```python
from build123d import *

# Parameters (mm, degrees)
SKETCH_1_R          = 1.65
EXTRUDE_1_DEPTH     = 3
SKETCH_3_W          = 62
SKETCH_3_H          = 11.5
EXTRUDE_2_DEPTH     = 3
FILLET_1_R          = 5
CUT_EXTRUDE_1_DEPTH = 10
SKETCH_4_R          = 4.5
SKETCH_4_R_2        = 1.75
EXTRUDE_3_DEPTH     = 3
FILLET_2_R          = 2
SKETCH_5_R          = 1.75
CUT_EXTRUDE_2_DEPTH = 3
SKETCH_6_OUTSIDE_W  = 115.11
SKETCH_6_OUTSIDE_H  = 116.61
CUT_EXTRUDE_4_DEPTH = 10
FILLET_3_R          = 5


with BuildPart() as part:
    # 草图1 → 凸台-拉伸1 (new body)
    with BuildSketch(Plane(origin=(0, 0, 0), x_dir=(1, 0, 0), z_dir=(0, 1, 0))):
        with BuildLine():
            Line((-42, 39), (42, 39))
            ThreePointArc((42, 39), (43.414213562, 38.414213562), (44, 37))
            Line((44, 37), (44, 33))
            ThreePointArc((44, 33), (43.414213562, 31.585786438), (42, 31))
            Line((42, 31), (33, 31))
            ThreePointArc((33, 31), (31.585786438, 30.414213562), (31, 29))
            Line((31, 29), (31, -29))
            ThreePointArc((31, -29), (31.585786438, -30.414213562), (33, -31))
            Line((33, -31), (42, -31))
            ThreePointArc((42, -31), (43.414213562, -31.585786438), (44, -33))
            Line((44, -33), (44, -37))
            ThreePointArc((44, -37), (43.414213562, -38.414213562), (42, -39))
            Line((42, -39), (-42, -39))
            ThreePointArc((-42, -39), (-43.414213562, -38.414213562), (-44, -37))
            Line((-44, -37), (-44, -33))
            ThreePointArc((-44, -33), (-43.414213562, -31.585786438), (-42, -31))
            Line((-42, -31), (-33, -31))
            ThreePointArc((-33, -31), (-31.585786438, -30.414213562), (-31, -29))
            Line((-31, -29), (-31, 29))
            ThreePointArc((-31, 29), (-31.585786438, 30.414213562), (-33, 31))
            Line((-33, 31), (-42, 31))
            ThreePointArc((-42, 31), (-43.414213562, 31.585786438), (-44, 33))
            Line((-44, 33), (-44, 37))
            ThreePointArc((-44, 37), (-43.414213562, 38.414213562), (-42, 39))
        make_face()
        with Locations(Location((-40, 35, 0), (0, 0, 270))):
            Circle(SKETCH_1_R, mode=Mode.SUBTRACT)
        with Locations(Location((40, 35, 0), (0, 0, 270))):
            Circle(SKETCH_1_R, mode=Mode.SUBTRACT)
        with Locations(Location((-40, -35, 0), (0, 0, 270))):
            Circle(SKETCH_1_R, mode=Mode.SUBTRACT)
        with Locations(Location((40, -35, 0), (0, 0, 270))):
            Circle(SKETCH_1_R, mode=Mode.SUBTRACT)
        with BuildLine():
            Line((-22.8, 30.1), (-26, 30.1))
            ThreePointArc((-26, 30.1), (-27, 29.1), (-26, 28.1))
            Line((-26, 28.1), (-26, 16.9))
            ThreePointArc((-26, 16.9), (-27, 15.9), (-26, 14.9))
            Line((-26, 14.9), (-22.8, 14.9))
            ThreePointArc((-22.8, 14.9), (-21.8, 15.9), (-22.8, 16.9))
            Line((-22.8, 16.9), (-22.8, 28.1))
            ThreePointArc((-22.8, 28.1), (-21.8, 29.1), (-22.8, 30.1))
        make_face(mode=Mode.SUBTRACT)
        with BuildLine():
            Line((22.8, 30.1), (26, 30.1))
            ThreePointArc((26, 30.1), (27, 29.1), (26, 28.1))
            Line((26, 28.1), (26, 16.9))
            ThreePointArc((26, 16.9), (27, 15.9), (26, 14.9))
            Line((26, 14.9), (22.8, 14.9))
            ThreePointArc((22.8, 14.9), (21.8, 15.9), (22.8, 16.9))
            Line((22.8, 16.9), (22.8, 28.1))
            ThreePointArc((22.8, 28.1), (21.8, 29.1), (22.8, 30.1))
        make_face(mode=Mode.SUBTRACT)
        with BuildLine():
            Line((22.8, -30.1), (26, -30.1))
            ThreePointArc((26, -30.1), (27, -29.1), (26, -28.1))
            Line((26, -28.1), (26, -16.9))
            ThreePointArc((26, -16.9), (27, -15.9), (26, -14.9))
            Line((26, -14.9), (22.8, -14.9))
            ThreePointArc((22.8, -14.9), (21.8, -15.9), (22.8, -16.9))
            Line((22.8, -16.9), (22.8, -28.1))
            ThreePointArc((22.8, -28.1), (21.8, -29.1), (22.8, -30.1))
        make_face(mode=Mode.SUBTRACT)
        with BuildLine():
            Line((-22.8, -30.1), (-26, -30.1))
            ThreePointArc((-26, -30.1), (-27, -29.1), (-26, -28.1))
            Line((-26, -28.1), (-26, -16.9))
            ThreePointArc((-26, -16.9), (-27, -15.9), (-26, -14.9))
            Line((-26, -14.9), (-22.8, -14.9))
            ThreePointArc((-22.8, -14.9), (-21.8, -15.9), (-22.8, -16.9))
            Line((-22.8, -16.9), (-22.8, -28.1))
            ThreePointArc((-22.8, -28.1), (-21.8, -29.1), (-22.8, -30.1))
        make_face(mode=Mode.SUBTRACT)
    extrude(amount=EXTRUDE_1_DEPTH)

    # 草图3 → 凸台-拉伸2 (add)
    with BuildSketch(Plane(origin=(0, 3, 0), x_dir=(1, 0, 0), z_dir=(0, 1, 0))):
        with Locations((0, 44.75)):
            Rectangle(SKETCH_3_W, SKETCH_3_H)
    extrude(amount=-EXTRUDE_2_DEPTH)

    # 圆角1
    fillet_1_edges = [part.edges().sort_by_distance(p)[0] for p in [
        (31, 1.5, -50.5),
        (31, 1.5, -39),
        (-31, 1.5, -39),
        (-31, 1.5, -50.5),
    ]]
    fillet(fillet_1_edges, radius=FILLET_1_R)

    # 草图2 → 切除-拉伸1 (cut)
    with BuildSketch(Plane(origin=(0, 3, 0), x_dir=(1, 0, 0), z_dir=(0, 1, 0))):
        with BuildLine():
            Line((-1, 47.232050808), (-14, 39.726497308))
            ThreePointArc((-14, 39.726497308), (-14.732050808, 38.994446501), (-15, 37.994446501))
            Line((-15, 37.994446501), (-15, -3.21999191))
            ThreePointArc((-15, -3.21999191), (-14.111140466, -4.882931135), (-12.234633135, -5.067750975))
            Line((-12.234633135, -5.067750975), (0, 0))
            Line((0, 0), (12.234633135, -5.067750975))
            ThreePointArc((12.234633135, -5.067750975), (14.111140466, -4.882931135), (15, -3.21999191))
            Line((15, -3.21999191), (15, 37.994446501))
            ThreePointArc((15, 37.994446501), (14.732050808, 38.994446501), (14, 39.726497308))
            Line((14, 39.726497308), (1, 47.232050808))
            ThreePointArc((1, 47.232050808), (0, 47.5), (-1, 47.232050808))
        make_face()
        with BuildLine():
            Line((-0.765366865, -5.728986337), (-14.765366865, -11.52797621))
            ThreePointArc((-14.765366865, -11.52797621), (-15.662939225, -12.264594809), (-16, -13.375735275))
            Line((-16, -13.375735275), (-16, -17.705304076))
            ThreePointArc((-16, -17.705304076), (-15.111140466, -19.368243301), (-13.234633135, -19.553063141))
            Line((-13.234633135, -19.553063141), (0, -14.071098604))
            Line((0, -14.071098604), (13.234633135, -19.553063141))
            ThreePointArc((13.234633135, -19.553063141), (15.111140466, -19.368243301), (16, -17.705304076))
            Line((16, -17.705304076), (16, -13.375735275))
            ThreePointArc((16, -13.375735275), (15.662939225, -12.264594809), (14.765366865, -11.52797621))
            Line((14.765366865, -11.52797621), (0.765366865, -5.728986337))
            ThreePointArc((0.765366865, -5.728986337), (0, -5.576745402), (-0.765366865, -5.728986337))
        make_face()
        with BuildLine():
            Line((14.765366865, -26.52797621), (0.765366865, -20.728986337))
            ThreePointArc((0.765366865, -20.728986337), (0, -20.576745402), (-0.765366865, -20.728986337))
            Line((-0.765366865, -20.728986337), (-14.765366865, -26.52797621))
            ThreePointArc((-14.765366865, -26.52797621), (-15.662939225, -27.264594809), (-16, -28.375735275))
            Line((-16, -28.375735275), (-16, -32.705304076))
            ThreePointArc((-16, -32.705304076), (-15.111140466, -34.368243301), (-13.234633135, -34.553063141))
            Line((-13.234633135, -34.553063141), (0, -29.071098604))
            Line((0, -29.071098604), (13.234633135, -34.553063141))
            ThreePointArc((13.234633135, -34.553063141), (15.111140466, -34.368243301), (16, -32.705304076))
            Line((16, -32.705304076), (16, -28.375735275))
            ThreePointArc((16, -28.375735275), (15.662939225, -27.264594809), (14.765366865, -26.52797621))
        make_face()
    extrude(amount=-CUT_EXTRUDE_1_DEPTH, mode=Mode.SUBTRACT)

    # 草图4 → 凸台-拉伸3 (add)
    # profile 1 of 4: a face of its own
    with BuildSketch(Plane(origin=(0, 3, 0), x_dir=(1, 0, 0), z_dir=(0, 1, 0))):
        with Locations((-32, 22.5)):
            Circle(SKETCH_4_R)
        with Locations((-32, 22.5)):
            Circle(SKETCH_4_R_2, mode=Mode.SUBTRACT)
    # profile 2 of 4: a face of its own
    with BuildSketch(Plane(origin=(0, 3, 0), x_dir=(1, 0, 0), z_dir=(0, 1, 0))):
        with Locations((32, 22.5)):
            Circle(SKETCH_4_R)
        with Locations((32, 22.5)):
            Circle(SKETCH_4_R_2, mode=Mode.SUBTRACT)
    # profile 3 of 4: a face of its own
    with BuildSketch(Plane(origin=(0, 3, 0), x_dir=(1, 0, 0), z_dir=(0, 1, 0))):
        with Locations((32, -22.5)):
            Circle(SKETCH_4_R)
        with Locations((32, -22.5)):
            Circle(SKETCH_4_R_2, mode=Mode.SUBTRACT)
    # profile 4 of 4: a face of its own
    with BuildSketch(Plane(origin=(0, 3, 0), x_dir=(1, 0, 0), z_dir=(0, 1, 0))):
        with Locations((-32, -22.5)):
            Circle(SKETCH_4_R)
        with Locations((-32, -22.5)):
            Circle(SKETCH_4_R_2, mode=Mode.SUBTRACT)
    extrude(amount=-EXTRUDE_3_DEPTH)

    # 圆角2
    fillet_2_edges = [part.edges().sort_by_distance(p)[0] for p in [
        (-31, 1.5, -18.112517806),
        (-31, 1.5, -26.887482194),
        (31, 1.5, -26.887482194),
        (31, 1.5, -18.112517806),
        (31, 1.5, 26.887482194),
        (31, 1.5, 18.112517806),
        (-31, 1.5, 26.887482194),
        (-31, 1.5, 18.112517806),
    ]]
    fillet(fillet_2_edges, radius=FILLET_2_R)

    # 草图5 → 切除-拉伸2 (cut)
    with BuildSketch(Plane(origin=(0, 3, 0), x_dir=(1, 0, 0), z_dir=(0, 1, 0))):
        with Locations(Location((-32, 22.5, 0), (0, 0, 270))):
            Circle(SKETCH_5_R)
        with Locations(Location((32, 22.5, 0), (0, 0, 270))):
            Circle(SKETCH_5_R)
        with Locations(Location((32, -22.5, 0), (0, 0, 270))):
            Circle(SKETCH_5_R)
        with Locations(Location((-32, -22.5, 0), (0, 0, 270))):
            Circle(SKETCH_5_R)
    extrude(amount=-CUT_EXTRUDE_2_DEPTH, mode=Mode.SUBTRACT)

    # 草图6 outside → 切除-拉伸4 (cut)
    with BuildSketch(Plane(origin=(0, 3, 0), x_dir=(1, 0, 0), z_dir=(0, 1, 0))):
        with Locations((0, 5.75)):
            Rectangle(SKETCH_6_OUTSIDE_W, SKETCH_6_OUTSIDE_H)
        Polygon((-31, 45.5), (-31, 28.922616289), (-44.52716968, 28.922616289), (-44.52716968, -29), (-31, -29), (-31, -39), (31, -39), (31, -28.922616289), (42.852208754, -28.922616289), (42.852208754, 29), (31, 29), (31, 45.5), (31, 52.188575174), (-31, 52.188575174), align=None, mode=Mode.SUBTRACT)
    extrude(amount=-CUT_EXTRUDE_4_DEPTH, mode=Mode.SUBTRACT)

    # 圆角3
    fillet_3_edges = [part.edges().sort_by_distance(p)[0] for p in [
        (-31, 1.5, 39),
        (31, 1.5, 39),
    ]]
    fillet(fillet_3_edges, radius=FILLET_3_R)


solid = part.part
```
Build history of the part. All positions in model axes, mm. A direction names the side the tool comes from. Coordinates: 2 decimals unless noted, no trailing zeros. Order: outer loops, then holes, each group sorted by start corner. A loop starts at its lowest first (then second) coordinate and runs counter-clockwise, first axis right, second up. Notation, with made-up numbers: M -31,0 L 15,0 A12 cw 15,17 Z; hole C 63,-4.5 d8. An arc over 180 degrees is marked long. One line per question, with ' | ' between items. Start each with the question number.
1. Mould opens along X. For faces 4 (the face through (29.5, 1.48, -49.07)), 5 (the face through (-6.71, 1.52, 16.85)), 6 (the face through (-1, 3, 4)) say: +X half, -X half, draft (parallel to the pull), parting line (faces both ways), or undercut.
2. Cut at B-B (x = 7.5). Write the cut outline in (y, z), plus the area to 3 significant figures.
3. Flat gauge pins, fed straight in: P1, Ø1.5, axis at y = 1.5, z = -21.5, coming from the -X side; P2, Ø1.5, axis at y = 1.5, z = -21.5, coming from the +X side. Where does each tip first touch, or does it go through?
4. Cut at D-D (z = 22.5). Write the cut outline in (x, y), plus the area to 3 significant figures.
5. Cut at C-C (z = -42). Write the cut outline in (x, y), plus the area to 3 significant figures.
6. Wall check: line 1 along X through (y, z) = (1.75, -22.5); line 2 along Z through (x, y) = (10.5, 1.7); line 3 along X through (y, z) = (0.95, 22.5). Give the ranges that are in metal, low to high. Write a range as [from, to].
7. Cut at A-A (z = -22.5). Write the cut outline in (x, y), plus the area to 3 significant figures.
8. Tool access for faces 1 (the face through (21.8, 1.5, 29.1)), 2 (the face through (-31, 2, -37)), 3 (the face through (31.5, 1.5, -17.4)): list every direction of +Z, -Z, +X, -X, +Y, -Y with a clear straight run to the whole face (end or side of a thin tool).
The answers:
1) face 4: +X half | face 5: undercut | face 6: draft
2) outline: M 0,-50.5 L 3,-50.5 L 3,-43.48 L 0,-43.48 Z; M 0,3.11 L 3,3.11 L 3,8.52 L 0,8.52 Z; M 0,17.18 L 3,17.18 L 3,23.52 L 0,23.52 Z; M 0,32.18 L 3,32.18 L 3,39 L 0,39 Z | area: 76.8 mm2
3) P1: stops at x = -36.49 | P2: stops at x = 36.49
4) outline: M -36.5,0 L -33.75,0 L -33.75,3 L -36.5,3 Z; M -30.25,0 L -26,0 L -26,3 L -30.25,3 Z; M -22.8,0 L -5.04,0 L -5.04,3 L -22.8,3 Z; M 5.04,0 L 22.8,0 L 22.8,3 L 5.04,3 Z; M 26,0 L 30.25,0 L 30.25,3 L 26,3 Z; M 33.75,0 L 36.5,0 L 36.5,3 L 33.75,3 Z | area: 149 mm2
5) outline: M -31,0 L -10.06,0 L -10.06,3 L -31,3 Z; M 10.06,0 L 31,0 L 31,3 L 10.06,3 Z | area: 126 mm2
6) line 1: x = [-36.5, -33.75], [-30.25, -26], [-22.8, -15], [15, 22.8], [26, 30.25], [33.75, 36.5] | line 2: z = [-50.5, -41.75], [4.35, 9.76], [18.42, 24.76], [33.42, 39] | line 3: x = [-36.5, -33.75], [-30.25, -26], [-22.8, -5.04], [5.04, 22.8], [26, 30.25], [33.75, 36.5]
7) outline: M -36.5,0 L -33.75,0 L -33.75,3 L -36.5,3 Z; M -30.25,0 L -26,0 L -26,3 L -30.25,3 Z; M -22.8,0 L -15,0 L -15,3 L -22.8,3 Z; M 15,0 L 22.8,0 L 22.8,3 L 15,3 Z; M 26,0 L 30.25,0 L 30.25,3 L 26,3 Z; M 33.75,0 L 36.5,0 L 36.5,3 L 33.75,3 Z | area: 88.8 mm2
8) face 1: +Y, -Y | face 2: -Z, -X, +Y, -Y | face 3: +X, +Y, -Y
